```python
from build123d import *

# Parameters (mm, degrees)
SKETCH_W   = 420
SKETCH_H   = 127
SKETCH_R   = 15
SKETCH_R_2 = 14
PAD_DEPTH  = 14


with BuildPart() as part:
    # Sketch → Pad (new body)
    with BuildSketch(Plane.XY):
        with Locations((210, 63.5)):
            Rectangle(SKETCH_W, SKETCH_H)
        with Locations((50, 77)):
            Circle(SKETCH_R, mode=Mode.SUBTRACT)
        with Locations((100, 80)):
            Circle(SKETCH_R_2, mode=Mode.SUBTRACT)
        with Locations((132, 87)):
            Circle(SKETCH_R_2, mode=Mode.SUBTRACT)
        with Locations((164, 93)):
            Circle(SKETCH_R_2, mode=Mode.SUBTRACT)
        with Locations((196, 98)):
            Circle(SKETCH_R_2, mode=Mode.SUBTRACT)
        with Locations((100, 30)):
            Circle(SKETCH_R_2, mode=Mode.SUBTRACT)
        with Locations((132, 37)):
            Circle(SKETCH_R_2, mode=Mode.SUBTRACT)
        with Locations((164, 43)):
            Circle(SKETCH_R_2, mode=Mode.SUBTRACT)
        with Locations((196, 48)):
            Circle(SKETCH_R_2, mode=Mode.SUBTRACT)
        with Locations((246, 77)):
            Circle(SKETCH_R, mode=Mode.SUBTRACT)
        with Locations((296, 80)):
            Circle(SKETCH_R_2, mode=Mode.SUBTRACT)
        with Locations((328, 87)):
            Circle(SKETCH_R_2, mode=Mode.SUBTRACT)
        with Locations((360, 93)):
            Circle(SKETCH_R_2, mode=Mode.SUBTRACT)
        with Locations((392, 98)):
            Circle(SKETCH_R_2, mode=Mode.SUBTRACT)
        with Locations((392, 48)):
            Circle(SKETCH_R_2, mode=Mode.SUBTRACT)
        with Locations((360, 43)):
            Circle(SKETCH_R_2, mode=Mode.SUBTRACT)
        with Locations((328, 37)):
            Circle(SKETCH_R_2, mode=Mode.SUBTRACT)
        with Locations((296, 30)):
            Circle(SKETCH_R_2, mode=Mode.SUBTRACT)
    extrude(amount=PAD_DEPTH)


solid = part.part
```
Here's how the part is built. I have some questions about the finished solid (model axes, mm). Give positions to 0.01 mm unless a question says otherwise; leave off trailing zeros. Loops run counter-clockwise (first coordinate to the right, second up) from the corner with the lowest first, then second, coordinate; pieces in that order, holes last. Notation, with made-up numbers: M 42,-12.75 L 64,-12.75 A20 ccw 64,24.25 Z; hole C 55,-25 d2. An arc over 180 degrees is marked long. Use one line per item in the form item = value. Start each with the question number.
Q1. Thinking about a two-plate mould opening in X: for faces 1 (the flat face through (207, 0, 7)), 2 (the cylindrical face through (182.014, 98.616, 6.902)), which applies, +X half, -X half, draft (parallel to the pull), parting line (faces both ways), or undercut?
Q2. If we section it at C-C (z = 3): State how many separate pieces and enclosed holes the cut face has, then the cut area to 3 significant figures.
Q3. Will this pin go through, and if not, where does the flat tip stop? pin 1 Ø17 at (x, y) = (360, 43) entering from +Z.
Q4. If we section it at D-D (x = 125): Write out the boundary of the cut face in (y, z), then the cut area to 3 significant figures.
Q5. If we section it at A-A (x = 328): Write out the boundary of the cut face in (y, z), then the cut area to 3 significant figures.
Q6. If we section it at B-B (x = 246): Write out the boundary of the cut face in (y, z).
Q7. I need wall thicknesses on line 1 along Y through (x, z) = (100, 5.25); line 2 along Y through (x, z) = (392, 3.5); line 3 along X through (y, z) = (70, 8.25). Which ranges of each line are inside material? Lowest first, please.
Taken from the geometry:
q1.face_1 = draft
q1.face_2 = undercut
q2.separate_pieces = 1
q2.enclosed_holes = 18
q2.area = 42,100 mm^2
q3.pin_1 = through
q4.outline = M 0,0 L 24.88,0 L 24.88,14 L 0,14 Z; M 49.12,0 L 74.88,0 L 74.88,14 L 49.12,14 Z; M 99.12,0 L 127,0 L 127,14 L 99.12,14 Z
q4.area = 1,100 mm^2
q5.outline = M 0,0 L 23,0 L 23,14 L 0,14 Z; M 51,0 L 73,0 L 73,14 L 51,14 Z; M 101,0 L 127,0 L 127,14 L 101,14 Z
q5.area = 994 mm^2
q6.outline = M 0,0 L 62,0 L 62,14 L 0,14 Z; M 92,0 L 127,0 L 127,14 L 92,14 Z
q7.line_1 = 0 to 16, 44 to 66, 94 to 127
q7.line_2 = 0 to 34, 62 to 84, 112 to 127
q7.line_3 = 0 to 36.73, 63.27 to 90.2, 109.8 to 232.73, 259.27 to 286.2, 305.8 to 420
